For this review, take the finished solid that the model builds, in its own axes (mm). A direction names the side the tool comes from. Coordinates: 2 decimals unless noted, no trailing zeros. Order: outer loops, then holes, each group sorted by start corner. A loop starts at its lowest first (then second) coordinate and runs counter-clockwise, first axis right, second up.
from build123d import *

# Parameters (mm, degrees)
SKETCH_1_R          = 5
EXTRUDE_1_DEPTH     = 4
SKETCH_4_R          = 7.5
CUT_EXTRUDE_3_DEPTH = 3
CUT_EXTRUDE_4_REACH = 6


with BuildPart() as part:
    # 草图1 → 凸台-拉伸1 (new body)
    with BuildSketch(Plane.XY):
        with BuildLine():
            Line((0, 12.25), (100, 12.25))
            ThreePointArc((100, 12.25), (112.25, 0), (100, -12.25))
            Line((100, -12.25), (0, -12.25))
            ThreePointArc((0, -12.25), (-12.25, 0), (0, 12.25))
        make_face()
        Circle(SKETCH_1_R, mode=Mode.SUBTRACT)
        with Locations((100, 0)):
            Circle(SKETCH_1_R, mode=Mode.SUBTRACT)
    extrude(amount=EXTRUDE_1_DEPTH)

    # 草图4 → 切除-拉伸3 (cut)
    with BuildSketch(Plane.XY.offset(2)):
        Circle(SKETCH_4_R)
        with Locations((100, 0)):
            Circle(SKETCH_4_R)
    extrude(amount=-CUT_EXTRUDE_3_DEPTH, mode=Mode.SUBTRACT)

    # 草图5 → 切除-拉伸4 (cut, up to next)
    with BuildSketch(Plane(origin=(0, 0, 0), x_dir=(-1, 0, 0), z_dir=(0, 0, -1)), mode=Mode.PRIVATE) as cut_extrude_4_sk1:
        with BuildLine():
            Line((-73, 7.5), (-87.516221291, -3.928572043))
            ThreePointArc((-87.516221291, -3.928572043), (-88.168863565, -6.15465414), (-86.279041363, -7.5))
            Line((-86.279041363, -7.5), (-58.092346966, -7.5))
            ThreePointArc((-58.092346966, -7.5), (-56.186421499, -6.106174988), (-56.937022619, -3.867448116))
            Line((-56.937022619, -3.867448116), (-73, 7.5))
        make_face()
    cut_extrude_4_tool1 = extrude(cut_extrude_4_sk1.sketch, amount=-CUT_EXTRUDE_4_REACH, mode=Mode.PRIVATE) & part.part
    add(cut_extrude_4_tool1.solids().sort_by_distance((72.350084, -2.302404, 0))[0], mode=Mode.SUBTRACT)
    # 草图5 → 切除-拉伸4 (cut, up to next)
    with BuildSketch(Plane(origin=(0, 0, 0), x_dir=(-1, 0, 0), z_dir=(0, 0, -1)), mode=Mode.PRIVATE) as cut_extrude_4_sk2:
        with BuildLine():
            Line((-32, -7.5), (-17.483778709, 3.928572043))
            ThreePointArc((-17.483778709, 3.928572043), (-16.831136435, 6.15465414), (-18.720958637, 7.5))
            Line((-18.720958637, 7.5), (-46.907653034, 7.5))
            ThreePointArc((-46.907653034, 7.5), (-48.813578501, 6.106174988), (-48.062977381, 3.867448116))
            Line((-48.062977381, 3.867448116), (-32, -7.5))
        make_face()
    cut_extrude_4_tool2 = extrude(cut_extrude_4_sk2.sketch, amount=-CUT_EXTRUDE_4_REACH, mode=Mode.PRIVATE) & part.part
    add(cut_extrude_4_tool2.solids().sort_by_distance((32.649916, 2.302404, 0))[0], mode=Mode.SUBTRACT)


solid = part.part
1. To check wall thickness, follow L1, parallel to X at y = 1, z = 1.7; L2, parallel to Y at x = 0, z = 2.85; L3, parallel to Y at x = 0, z = 1.5. State the ranges of each line that lie inside material, in increasing order.
Answer below:
L1: x = -12.21 to -7.43, 7.43 to 21.2, 44.01 to 63.82, 81.26 to 92.57, 107.43 to 112.21
L2: y = -12.25 to -5, 5 to 12.25
L3: y = -12.25 to -7.5, 7.5 to 12.25
2. Clearance check with flat-ended pins moving along their axes: pin 1 Ø5 at (x, y) = (14.5, -8.5) entering from -Z; pin 2 Ø7.5 at (x, y) = (3, -2) entering from -Z. State where each tip first meets the part, or that it passes through.
Answer below:
pin 1: stops at z = 0
pin 2: stops at z = 2
3. Take a section at D-D, the plane y = -6.25. Give the boundary of the cut face in (x, z), plus the area to 3 significant figures.
Answer below:
outline: (-10.54, 0) - (-4.15, 0) - (-4.15, 2) - (4.15, 2) - (4.15, 0) - (30.41, 0) - (30.41, 4) - (-10.54, 4) - close; (33.77, 0) - (56.24, 0) - (56.24, 4) - (33.77, 4) - close; (88.13, 0) - (95.85, 0) - (95.85, 2) - (104.15, 2) - (104.15, 0) - (110.54, 0) - (110.54, 4) - (88.13, 4) - close
area: 310 mm2
4. Take a section at B-B, the plane y = 1.75. Give the boundary of the cut face in (x, z), plus the area to 3 significant figures.
Answer below:
outline: (-12.12, 0) - (-7.29, 0) - (-7.29, 2) - (-4.68, 2) - (-4.68, 4) - (-12.12, 4) - close; (4.68, 2) - (7.29, 2) - (7.29, 0) - (20.25, 0) - (20.25, 4) - (4.68, 4) - close; (45.07, 0) - (64.87, 0) - (64.87, 4) - (45.07, 4) - close; (80.3, 0) - (92.71, 0) - (92.71, 2) - (95.32, 2) - (95.32, 4) - (80.3, 4) - close; (104.68, 2) - (107.29, 2) - (107.29, 0) - (112.12, 0) - (112.12, 4) - (104.68, 4) - close
area: 240 mm2
5. Machinability: for faces 1 (the face through (112.247, 0.269, 1.972)), 2 (the face through (40.14, -1.74, 1.97)), 3 (the face through (-7.493, 0.33, 1.014)), which of the approach directions +Z, -Z, +X, -X, +Y, -Y give a long, thin tool a straight path to every point of the face, cutting with its end or side? Answer none if there is none.
Answer below:
face 1: +Z, -Z, +X
face 2: +Z, -Z
face 3: -Z
6. The part is to be moulded in two halves that separate along X. For faces 4 (the face through (48.803, 6.14, 1.972)), 5 (the face through (51, -12.25, 2)), 6 (the face through (-12.247, -0.269, 1.972)), say which applies: +X half, -X half, draft (parallel to the pull), parting line (faces both ways), or undercut.
Answer below:
face 4: undercut
face 5: draft
face 6: -X half
7. Take a section at C-C, the plane x = 77. Give the boundary of the cut face in (y, z).
Answer below:
outline: (-12.25, 0) - (-7.5, 0) - (-7.5, 4) - (-12.25, 4) - close; (4.35, 0) - (12.25, 0) - (12.25, 4) - (4.35, 4) - close
8. Take a section at A-A, the plane z = 3.4. Give the boundary of the cut face in (x, y), plus the area to 3 significant figures.
Answer below:
outline: (0, -12.25) - (100, -12.25) arc R12.25 ccw to (100, 12.25) - (0, 12.25) arc R12.25 ccw to start; hole circle Ø10 at (0, 0); hole (17.48, 3.93) - (32, -7.5) - (48.06, 3.87) arc R2 ccw to (46.91, 7.5) - (18.72, 7.5) arc R2 ccw to start; hole (56.94, -3.87) arc R2 ccw to (58.09, -7.5) - (86.28, -7.5) arc R2 ccw to (87.52, -3.93) - (73, 7.5) - close; hole circle Ø10 at (100, 0)
area: 2,190 mm2
